Model file for the job. Use its own axes, mm. A direction names the side the tool comes from. Coordinates: 2 decimals unless noted, no trailing zeros. Order: outer loops, then holes, each group sorted by start corner. A loop starts at its lowest first (then second) coordinate and runs counter-clockwise, first axis right, second up. Notation, with made-up numbers: (82.25, 84.5) -> (86.25, 84.5) arc R31 cw to (86.25, 123.5) -> close; hole circle Ø9 at (89, 5.5). An arc over 180 degrees is marked (long way). Return JSON: item names as keys, results as strings. Group by question number.
1) Cut at A-A (y = 12.75). Write the cut outline in (x, z), and give its area (3 significant figures).
2) Cut at B-B (x = 10). Write the cut outline in (y, z).
3) Flat gauge pins, fed straight in: pin 1 (1.8 mm diameter, centred on x = 14.5, z = -24.5, fed in from -Y); pin 2 (1 mm diameter, centred on x = -21.5, y = 9.5, fed in from +Z); pin 3 (5 mm diameter, centred on x = -9, y = 7.5, fed in from -Z); pin 4 (2.5 mm diameter, centred on x = 16.5, z = -24.5, fed in from +Y). Where does each tip first touch, or does it go through?
4) Which spindle directions (+Z, -Z, +X, -X, +Y, -Y) get a long thin tool onto all of the face, cutting with end or side? Do faces 1 (the flat face through (0, 8, 23.3)), 2 (the flat face through (0, -1, 23.3)), 3 (the flat face through (0, -1, -23.3)). Say none if no direction does.
5) Probe line 1 (Z direction, x = 24.5, y = 9.75); line 2 (Z direction, x = -9, y = 12). List the from-to ranges inside material, lowest first.
6) Cut at C-C (y = -1.75). Write the cut outline in (x, z).
Autodesk Inventor part; units mm, degrees
ref_plane "YZ Plane" through (0, 0, 0) normal (1, 0, 0) x (0, 1, 0)
ref_plane "XZ Plane" through (0, 0, 0) normal (0, 1, 0) x (-1, 0, 0)
ref_plane "XY Plane" through (0, 0, 0) normal (0, 0, 1) x (1, 0, 0)
sketch "Boceto1" plane through (0, 0, 0) normal (0, 1, 0) x (-1, 0, 0)
  line L0 (-34, 25.5) -> (34, 25.5)
  line L1 (34, 25.5) -> (34, -25.5)
  line L2 (34, -25.5) -> (-34, -25.5)
  line L3 (-34, -25.5) -> (-34, 25.5)
  line L4 (-34, 25.5) -> (34, -25.5) construction
  line L5 (34, 25.5) -> (-34, -25.5) construction
  point P0 (0, 0)
  dimension "d0" = 68
  dimension "d1" = 51
extrude "Extrusión1" add sketch "Boceto1" along normal blind 14
sketch "Boceto2" plane through (34, 0, 25.5) normal (1, 0, 0) x (0, 0, -1)
  line L0 (51, 0) -> (0, 0)
  line L1 (0, 0) -> (2.2, 0)
  line L2 (2.2, 0) -> (2.2, 1.7)
  line L3 (2.2, 1.7) -> (0, 1.7)
  line L4 (0, 1.7) -> (0, 0)
  line L5 (0, 0) -> (0, 14)
  line L6 (2.2, 1.7) -> (0, 1.7)
  line L7 (0, 1.7) -> (0, 14)
  line L8 (0, 14) -> (2.2, 14)
  line L9 (2.2, 14) -> (2.2, 1.7)
  line L10 (25.5, -2.8463) -> (25.5, 17.6313)
  line L11 (48.8, 1.7) -> (51, 1.7)
  line L12 (51, 0) -> (51, 14)
  line L13 (51, 14) -> (48.8, 14)
  line L14 (48.8, 14) -> (48.8, 1.7)
  point P0 (25.5, 0)
  dimension "d4" = 2.2
  dimension "d5" = 1.7
  dimension "d8" = 51
  dimension "d9" = 12.3
  dimension "d10" = 46.6
extrude "Extrusión2" cut sketch "Boceto2" against normal through all contours L11 L14 L13 L12 | L3 L5 L8 L9
sketch "Boceto3" plane through (34, 1.7, -23.3) normal (0, 0, -1) x (-1, 0, 0)
  line L0 (68, 12.3) -> (0, 12.3)
  line L1 (0, 0) -> (68, 0)
  line L2 (0, 12.3) -> (34, 12.3)
  line L3 (34, 12.3) -> (34, 0)
  line L4 (34, 0) -> (0, 0)
  line L5 (0, 0) -> (0, 12.3)
  line L6 (68, 0) -> (68, 12.3)
  line L7 (68, 12.3) -> (34, 12.3)
  line L8 (34, 12.3) -> (34, 5.1984)
  line L9 (34, 5.1984) -> (68, 5.1984)
  line L10 (68, 5.1984) -> (68, 12.3)
  line L11 (34, 12.3) -> (23.5366, 12.3)
  line L12 (23.5366, 12.3) -> (28.5366, 12.3)
  line L13 (28.5366, 12.3) -> (43.5366, 12.3)
  line L14 (28.5366, 12.3) -> (43.5366, 12.3)
  line L15 (43.5366, 12.3) -> (43.5366, 5.1984)
  line L16 (43.5366, 5.1984) -> (28.5366, 5.1984)
  line L17 (28.5366, 5.1984) -> (28.5366, 12.3)
  point P0 (34, -1.7)
  point P1 (43.5366, 12.3)
  point P2 (28.5366, 12.3)
  point P3 (34, 5.1984)
  dimension "d11" = 34
  dimension "d12" = 5
  dimension "d13" = 15
extrude "Extrusión3" add sketch "Boceto3" along normal blind 1 contours L15 L9 L3 L0 | L3 L16 L17 L0
sketch "Boceto4" plane through (0, 0, 0) normal (0, -1, 0) x (1, 0, 0)
  line L0 (-34, 23.3) -> (34, 23.3)
  line L1 (-34, -23.3) -> (-34, 23.3)
  line L2 (34, 23.3) -> (-34, 23.3)
  line L3 (-9.5366, -23.3) -> (-34, -23.3)
  line L4 (-34, 23.3) -> (-34, -23.3)
  line L5 (34, 23.3) -> (34, -23.3)
  line L6 (-34, -23.3) -> (34, -23.3)
  line L7 (34, -23.3) -> (34, 23.3)
  point P0 (0, 0)
extrude "Extrusión4" add sketch "Boceto4" along normal blind 3
properties part number "PCB_Tamaño"
Answers below:
{
 "1": {"outline": "(-34, -23.3) -> (-9.54, -23.3) -> (-9.54, -24.3) -> (5.46, -24.3) -> (5.46, -23.3) -> (34, -23.3) -> (34, 23.3) -> (-34, 23.3) -> close", "area": "3,180 mm^2"},
 "2": {"outline": "(-3, -23.3) -> (0, -23.3) -> (0, -25.5) -> (1.7, -25.5) -> (1.7, -23.3) -> (14, -23.3) -> (14, 23.3) -> (1.7, 23.3) -> (1.7, 25.5) -> (0, 25.5) -> (0, 23.3) -> (-3, 23.3) -> close"},
 "3": {"pin 1": "stops at y = 0", "pin 2": "stops at z = 23.3", "pin 3": "stops at z = -24.3", "pin 4": "stops at y = 14"},
 "4": {"face 1": "+Z, +X, -X, +Y", "face 2": "+Z, +X, -X, -Y", "face 3": "-Z, +X, -X, -Y"},
 "5": {"line 1": "z = -23.3 to 23.3", "line 2": "z = -24.3 to 23.3"},
 "6": {"outline": "(-34, -23.3) -> (34, -23.3) -> (34, 23.3) -> (-34, 23.3) -> close"}
}
